Could you check a few things on this model? Use its own coordinates, in mm. Coordinates: 2 decimals unless noted, no trailing zeros. Order: outer loops, then holes, each group sorted by start corner. A loop starts at its lowest first (then second) coordinate and runs counter-clockwise, first axis right, second up. Notation, with made-up numbers: (-33.5, -6) - (-13.5, -6) arc R14 ccw to (-13.5, 7) - close; hole circle Ø5 at (-6.5, 57). An arc over 180 degrees is marked (long way). One line per item, written item: value.
from build123d import *

# Parameters (mm, degrees)
F0_W     = 550
F0_H     = 120
F0_R     = 7.5
F1_DEPTH = 25


with BuildPart() as f1:
    # F0 (on Front) → F1 (new body)
    with BuildSketch(Plane.XZ):
        with Locations((175, 0)):
            Rectangle(F0_W, F0_H)
        with Locations((-50, 0)):
            Circle(F0_R, mode=Mode.SUBTRACT)
        Circle(F0_R, mode=Mode.SUBTRACT)
        with Locations((50, 0)):
            Circle(F0_R, mode=Mode.SUBTRACT)
        with Locations((100, 0)):
            Circle(F0_R, mode=Mode.SUBTRACT)
        with Locations((150, 0)):
            Circle(F0_R, mode=Mode.SUBTRACT)
        with Locations((200, 0)):
            Circle(F0_R, mode=Mode.SUBTRACT)
        with Locations((250, 0)):
            Circle(F0_R, mode=Mode.SUBTRACT)
        with Locations((300, 0)):
            Circle(F0_R, mode=Mode.SUBTRACT)
        with Locations((350, 0)):
            Circle(F0_R, mode=Mode.SUBTRACT)
        with Locations((400, 0)):
            Circle(F0_R, mode=Mode.SUBTRACT)
    extrude(amount=F1_DEPTH)


solid = f1.part
Item 1: If I drill on probe 1 along Z at (x, y) = (-50, -8), over which ranges is the centre line in solid material (lowest first)?
Conclusion:
probe 1: -60 to -7.5, 7.5 to 60
Item 2: I'm going to push a flat-ended pin straight in: pin 1 Ø9 at (x, z) = (300, 0) entering from +Y. Where does the tip first touch, or does it pass through?
Conclusion:
pin 1: through
Item 3: I want a section at B-B on y = -15. Give the number of separate pieces and of enclosed holes in the cut face, then the cut area to 3 significant figures.
Conclusion:
separate pieces: 1
enclosed holes: 10
area: 64,200 mm²
Item 4: I want a section at A-A on x = 150. Please give me the cut outline in (y, z).
Conclusion:
outline: (-25, -60) - (0, -60) - (0, -7.5) - (-25, -7.5) - close; (-25, 7.5) - (0, 7.5) - (0, 60) - (-25, 60) - close
Item 5: Thinking about a two-plate mould opening in X: for faces 1 (the face through (-100, -12, -1)), 2 (the face through (450, -12, -1)), 3 (the face through (171, 0, 1)), 4 (the face through (256.93, -12.32, -2.87)), which applies, pulls with the +X half, pulls with the -X half, needs draft (parallel to the pull), parting line crosses it, or undercut?
Conclusion:
face 1: pulls with the -X half
face 2: pulls with the +X half
face 3: needs draft
face 4: undercut
